Drawing for the job (mm, zero at the part's lowest x, y, z). A direction names the side the tool comes from. Give positions to 0.01 mm unless a question says otherwise; leave off trailing zeros. Order: outer loops, then holes, each group sorted by start corner. A loop starts at its lowest first (then second) coordinate and runs counter-clockwise, first axis right, second up. Notation, with made-up numbers: (1.25, 1.5) - (60.25, 1.5) arc R18 cw to (60.25, 14.5) - close; hole circle Ø3 at (23.5, 67.5). An arc over 180 degrees is marked (long way). One line per item, written item: value.
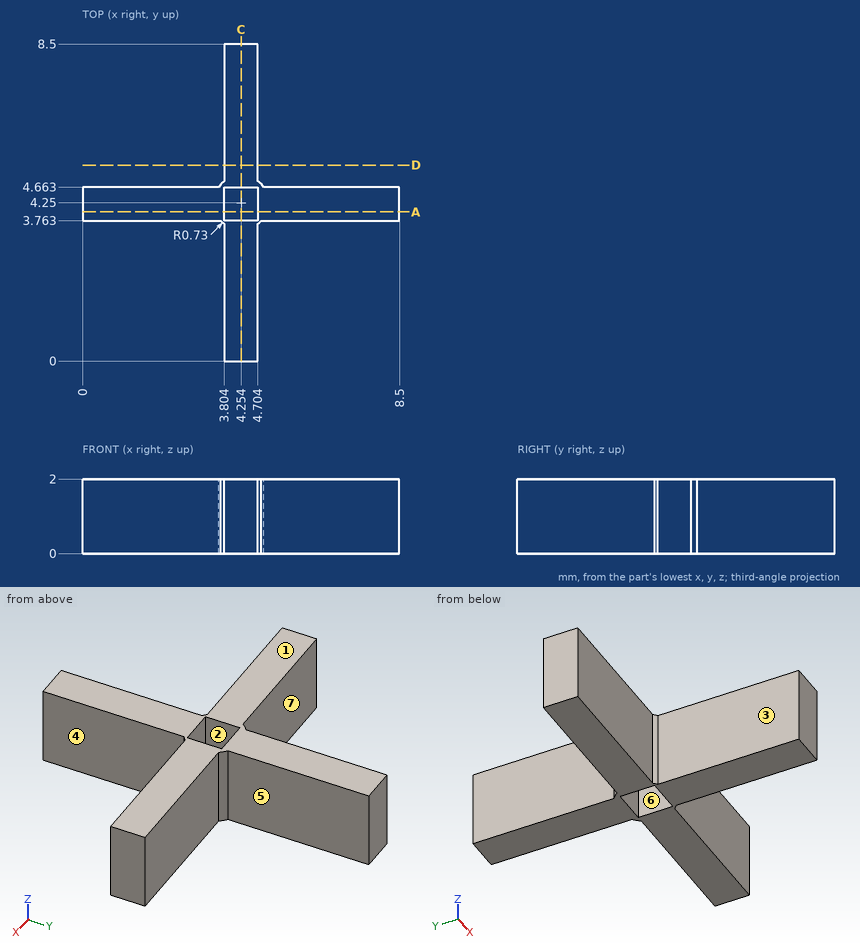
(1) Slice it at C-C, the plane x = 4.25. Give the cut face in (y, z).
Completed:
outline: (0, 0) - (3.76, 0) - (3.76, 2) - (0, 2) - close; (4.66, 0) - (8.5, 0) - (8.5, 2) - (4.66, 2) - close
(2) Drill centre lines: line 1 (X direction, y = 4, z = 0.8); line 2 (Y direction, x = 4.5, z = 0.1); line 3 (X direction, y = 2.25, z = 0.15). Where is each one in solid material? Low to high.
Completed:
line 1: 0 to 3.8, 4.7 to 8.5
line 2: 0 to 3.76, 4.66 to 8.5
line 3: 3.8 to 4.7
(3) Pin check, flat tips, straight feed: P1, Ø0.6, axis at x = 1.5, z = 0.5, coming from the +Y side; P2, Ø1, axis at y = 1, z = 0.5, coming from the +X side; P3, Ø1, axis at y = 6.5, z = 1, coming from the -X side. Stop position of each tip, or through.
Completed:
P1: y = 4.66
P2: x = 4.7
P3: x = 3.8
(4) Pull direction X, two halves, no side cores. Call the marked faces 1, 2 and 3: +X half, -X half, draft (parallel to the pull), parting line (faces both ways), or undercut.
Completed:
face 1: draft
face 2: undercut
face 3: -X half
(5) Slice it at D-D, the plane y = 5.25. Give the cut face in (x, z).
Completed:
outline: (3.8, 0) - (4.7, 0) - (4.7, 2) - (3.8, 2) - close
(6) Slice it at A-A, the plane y = 4. Give the cut face in (x, z).
Completed:
outline: (0, 0) - (3.8, 0) - (3.8, 2) - (0, 2) - close; (4.7, 0) - (8.5, 0) - (8.5, 2) - (4.7, 2) - close
(7) 3-axis set-ups, long thin cutter, end or side, ignore diameter. For the marked faces 4, 5, 6 and 7: which of +Z, -Z, +X, -X, +Y, -Y reach the whole face in a straight line?
Completed:
face 4: +Z, -Z, +X, -Y
face 5: +Z, -Z, +X, +Y
face 6: +Z, -Z
face 7: +Z, -Z, -X, +Y
